Build history of the part. All positions in model axes, mm. A direction names the side the tool comes from. Round coordinates to 2 decimals unless told otherwise and drop trailing zeros. Write each loop counter-clockwise with the first axis right and the second up, starting at its lowest first coordinate (ties: lowest second). Pieces come first, ordered by that corner, then holes.
Item 1: 3-axis set-ups, long thin cutter, end or side, ignore diameter. For faces 1 (the cylindrical face through (-0.596, -2.685, 3.374)), 2 (the cylindrical face through (-1.5, 0.07, 1.18)), 3 (the cylindrical face through (0.74, -3.32, -0.26)), 4 (the flat face through (7.5, 2.5, -0.5)), 5 (the flat face through (3.5, 1.4, -1.25)): which of +Z, -Z, +X, -X, +Y, -Y reach the whole face in a straight line?
Item 2: Band-saw the part on A-A, the plane z = -0.5. Write the cut outline in (x, y).
Item 3: Drop flat-ended pins along their axis: pin 1 Ø4.5 at (x, y) = (1, -1) entering from +Z; pin 2 Ø1.5 at (x, y) = (10, -1) entering from -Z; pin 3 Ø1 at (x, z) = (8, -0.5) entering from +Y; pin 4 Ø2 at (x, z) = (25, 0) entering from -Y. Give the stop position or say it passes through.
Item 4: Mould opens along X. For faces 6 (the flat face through (6.464, 0, -1)), 7 (the flat face through (19, 0, 2.6)), 8 (the flat face through (-1.5, -0.7, 0.75)) say: +X half, -X half, draft (parallel to the pull), parting line (faces both ways), or undercut.
Item 5: Band-saw the part on B-B, the plane x = 14.5. Write the cut outline in (y, z), then the cut area to 3 significant figures.
Item 6: Wall check: probe 1 along Z at (x, y) = (6.5, 0.25); probe 2 along Z at (x, y) = (25.5, 0.5); probe 3 along X at (y, z) = (-1.75, 2.25). Give the ranges that are in metal, low to high.
Item 7: Band-saw the part on C-C, the plane x = 20.7. Write the cut outline in (y, z), then the cut area to 3 significant figures.
```python
from build123d import *

# Parameters (mm, degrees)
BOSS_EXTRUDE1_DEPTH = 2.6
SKETCH2_R           = 4.75
BOSS_EXTRUDE2_DEPTH = 2.5
SKETCH3_R           = 2.5
CUT_EXTRUDE1_DEPTH  = 4
SKETCH4_R           = 0.75
CUT_EXTRUDE2_DEPTH  = 4
SKETCH5_R           = 4.75
BOSS_EXTRUDE3_DEPTH = 1.25
CHAMFER1_SIZE       = 2
CHAMFER1_SIZE2      = 1.154700538
BOSS_EXTRUDE4_DEPTH = 1.25
CHAMFER2_SIZE       = 2
CHAMFER2_SIZE2      = 1.154700538
SKETCH7_W           = 3
SKETCH7_H           = 5
CUT_EXTRUDE3_DEPTH  = 1.25
SKETCH8_R           = 2.75
CUT_EXTRUDE4_DEPTH  = 3.5
SKETCH9_R           = 3.4
CUT_EXTRUDE5_DEPTH  = 2
CHAMFER3_SIZE       = 0.5
SKETCH10_R          = 1.5
CUT_EXTRUDE6_DEPTH  = 5


with BuildPart() as part:
    # Sketch1 → Boss-Extrude1 (new body)
    with BuildSketch(Plane.XY):
        with BuildLine():
            Line((1.009697661, 5.914432402), (29.5, 3.5))
            ThreePointArc((29.5, 3.5), (33, 0), (29.5, -3.5))
            Line((29.5, -3.5), (1.009697661, -5.914432402))
            ThreePointArc((1.009697661, -5.914432402), (-6, 0), (1.009697661, 5.914432402))
        make_face()
    extrude(amount=BOSS_EXTRUDE1_DEPTH)

    # Sketch2 → Boss-Extrude2 (add)
    with BuildSketch(Plane.XY.offset(2.6)):
        Circle(SKETCH2_R)
    extrude(amount=BOSS_EXTRUDE2_DEPTH)

    # Sketch3 → Cut-Extrude1 (cut)
    with BuildSketch(Plane.XY.offset(2.6)):
        Circle(SKETCH3_R)
    extrude(amount=CUT_EXTRUDE1_DEPTH, mode=Mode.SUBTRACT)

    # Sketch4 → Cut-Extrude2 (cut)
    with BuildSketch(Plane.XY.offset(2.6)):
        with Locations((30, 0)):
            Circle(SKETCH4_R)
        with Locations((26.9, 0)):
            Circle(SKETCH4_R)
        with Locations((23.8, 0)):
            Circle(SKETCH4_R)
        with Locations((20.7, 0)):
            Circle(SKETCH4_R)
        with Locations((17.6, 0)):
            Circle(SKETCH4_R)
        with Locations((14.5, 0)):
            Circle(SKETCH4_R)
    extrude(amount=-CUT_EXTRUDE2_DEPTH, mode=Mode.SUBTRACT)

    # Sketch5 → Boss-Extrude3 (add)
    with BuildSketch(Plane.XY.offset(2.6)):
        with BuildLine():
            Line((1.009697661, 5.914432402), (0, 6))
            ThreePointArc((0, 6), (-5.978569829, -0.50665846), (1.009697661, -5.914432402))
            Line((1.009697661, -5.914432402), (9, -5.237288136))
            Line((9, -5.237288136), (9, 5.237288136))
            Line((9, 5.237288136), (1.009697661, 5.914432402))
        make_face()
        Circle(SKETCH5_R, mode=Mode.SUBTRACT)
    extrude(amount=BOSS_EXTRUDE3_DEPTH)

    # Chamfer1
    chamfer1_edges = [part.edges().sort_by_distance(p)[0] for p in [
        (9, 0, 3.85),
    ]]
    chamfer1_side = [part.faces().sort_by_distance(p)[0] for p in [
        (4.988627845, -5.384452642, 3.85),
    ]]
    chamfer(chamfer1_edges, length=CHAMFER1_SIZE, length2=CHAMFER1_SIZE2, reference=chamfer1_side[0])

    # Sketch6 → Boss-Extrude4 (add)
    with BuildSketch(Plane(origin=(0, 0, 0), x_dir=(-1, 0, 0), z_dir=(0, 0, -1))):
        with BuildLine():
            Line((-1.009697661, -5.914432402), (0, -6))
            ThreePointArc((0, -6), (6, 0), (0, 6))
            Line((0, 6), (-1.009697661, 5.914432402))
            Line((-1.009697661, 5.914432402), (-9, 5.237288136))
            Line((-9, 5.237288136), (-9, -5.237288136))
            Line((-9, -5.237288136), (-1.009697661, -5.914432402))
        make_face()
    extrude(amount=BOSS_EXTRUDE4_DEPTH)

    # Chamfer2
    chamfer2_edges = [part.edges().sort_by_distance(p)[0] for p in [
        (9, 0, -1.25),
    ]]
    chamfer2_side = [part.faces().sort_by_distance(p)[0] for p in [
        (1.907695527, 0, -1.25),
    ]]
    chamfer(chamfer2_edges, length=CHAMFER2_SIZE, length2=CHAMFER2_SIZE2, reference=chamfer2_side[0])

    # Sketch7 → Cut-Extrude3 (cut)
    with BuildSketch(Plane(origin=(0, 0, -1.25), x_dir=(-1, 0, 0), z_dir=(0, 0, -1))):
        with Locations((-7.964462138, 0)):
            Rectangle(SKETCH7_W, SKETCH7_H)
    extrude(amount=-CUT_EXTRUDE3_DEPTH, mode=Mode.SUBTRACT)

    # Sketch8 → Cut-Extrude4 (cut)
    with BuildSketch(Plane.XY.offset(5.1)):
        Circle(SKETCH8_R)
    extrude(amount=-CUT_EXTRUDE4_DEPTH, mode=Mode.SUBTRACT)

    # Sketch9 → Cut-Extrude5 (cut)
    with BuildSketch(Plane(origin=(0, 0, -1.25), x_dir=(-1, 0, 0), z_dir=(0, 0, -1))):
        Circle(SKETCH9_R)
    extrude(amount=-CUT_EXTRUDE5_DEPTH, mode=Mode.SUBTRACT)

    # Chamfer3
    chamfer3_edges = [part.edges().sort_by_distance(p)[0] for p in [
        (-4.75, 0, 5.1),
    ]]
    chamfer(chamfer3_edges, length=CHAMFER3_SIZE)

    # Sketch10 → Cut-Extrude6 (cut)
    with BuildSketch(Plane.XY.offset(1.6)):
        Circle(SKETCH10_R)
    extrude(amount=-CUT_EXTRUDE6_DEPTH, mode=Mode.SUBTRACT)


solid = part.part
```
Results:
1. face 1: +Z
1. face 2: +Z, -Z
1. face 3: -Z
1. face 4: -Z, +X
1. face 5: -Z, +X, -X, +Y, -Y
2. outline: (0, -6) - (8.3, -5.3) - (8.3, -2.5) - (6.46, -2.5) - (6.46, 2.5) - (8.3, 2.5) - (8.3, 5.3) - (0, 6) arc R6 ccw to start; hole circle Ø6.8 at (0, 0)
3. pin 1: stops at z = 5.1
3. pin 2: stops at z = 0
3. pin 3: stops at y = 5.36
3. pin 4: stops at y = -3.97
4. face 6: +X half
4. face 7: draft
4. face 8: undercut
5. outline: (-4.77, 0) - (-0.75, 0) - (-0.75, 2.6) - (-4.77, 2.6) - close; (0.75, 0) - (4.77, 0) - (4.77, 2.6) - (0.75, 2.6) - close
5. area: 20.9 mm2
6. probe 1: z = 0 to 3.85
6. probe 2: z = 0 to 2.6
6. probe 3: x = -5.74 to -2.12, 2.12 to 32.53
7. outline: (-4.25, 0) - (-0.75, 0) - (-0.75, 2.6) - (-4.25, 2.6) - close; (0.75, 0) - (4.25, 0) - (4.25, 2.6) - (0.75, 2.6) - close
7. area: 18.2 mm2
